from build123d import *

# Parameters (mm, degrees)
BOSS_EXTRUDE1_DEPTH = 3
SKETCH6_W           = 10
SKETCH6_H           = 3
BOSS_EXTRUDE5_DEPTH = 25
SKETCH8_W           = 3
SKETCH8_H           = 10
BOSS_EXTRUDE7_DEPTH = 64.65
SKETCH9_W           = 10
SKETCH9_H           = 3
BOSS_EXTRUDE8_DEPTH = 115.212
SKETCH10_W          = 3
SKETCH10_H          = 22.5
BOSS_EXTRUDE9_DEPTH = 25
SKETCH11_R          = 4
CUT_EXTRUDE1_DEPTH  = 3


with BuildPart() as part:
    # Sketch2 → Boss-Extrude1 (new body)
    with BuildSketch(Plane(origin=(0, 0, 0), x_dir=(1, 0, 0), z_dir=(0, 1, 0))):
        with BuildLine():
            Line((26.055569119, 8.188046441), (26.055569119, -22.834953559))
            Line((26.055569119, -22.834953559), (-26.055569119, -22.834953559))
            Line((-26.055569119, -22.834953559), (-26.055569119, 8.188046441))
            ThreePointArc((-26.055569119, 8.188046441), (-21.514872246, 4.669726518), (-15.870079226, 5.73406431))
            ThreePointArc((-15.870079226, 5.73406431), (-10.616247764, 4.133629141), (-7, 0))
            ThreePointArc((-7, 0), (0, -7), (7, 0))
            ThreePointArc((7, 0), (10.616247764, 4.133629141), (15.870079226, 5.73406431))
            ThreePointArc((15.870079226, 5.73406431), (21.514872246, 4.669726518), (26.055569119, 8.188046441))
        make_face()
    extrude(amount=BOSS_EXTRUDE1_DEPTH)

    # Sketch6 → Boss-Extrude5 (add)
    with BuildSketch(Plane.XY.offset(22.834953559)):
        with Locations((-21.055569119, 1.5)):
            Rectangle(SKETCH6_W, SKETCH6_H)
    extrude(amount=BOSS_EXTRUDE5_DEPTH)

    # Sketch8 → Boss-Extrude7 (add)
    with BuildSketch(Plane(origin=(0, 0, 0), x_dir=(-1, 0, 0), z_dir=(0, -1, 0))):
        with Locations((24.555569119, -42.834953559)):
            Rectangle(SKETCH8_W, SKETCH8_H)
    extrude(amount=BOSS_EXTRUDE7_DEPTH)

    # Sketch9 → Boss-Extrude8 (add)
    with BuildSketch(Plane(origin=(-23.055569119, 0, 0), x_dir=(0, 0, -1), z_dir=(1, 0, 0))):
        with Locations((-42.834953559, -63.15)):
            Rectangle(SKETCH9_W, SKETCH9_H)
    extrude(amount=BOSS_EXTRUDE8_DEPTH)

    # Sketch10 → Boss-Extrude9 (add)
    with BuildSketch(Plane(origin=(0, -61.65, 0), x_dir=(1, 0, 0), z_dir=(0, 1, 0))):
        with Locations((90.656430881, -36.584953559)):
            Rectangle(SKETCH10_W, SKETCH10_H)
    extrude(amount=BOSS_EXTRUDE9_DEPTH)

    # Sketch11 → Cut-Extrude1 (cut)
    with BuildSketch(Plane(origin=(92.156430881, 0, 0), x_dir=(0, 0, -1), z_dir=(1, 0, 0))):
        with Locations((-36.584953559, -49.15)):
            Circle(SKETCH11_R)
    extrude(amount=-CUT_EXTRUDE1_DEPTH, mode=Mode.SUBTRACT)


solid = part.part
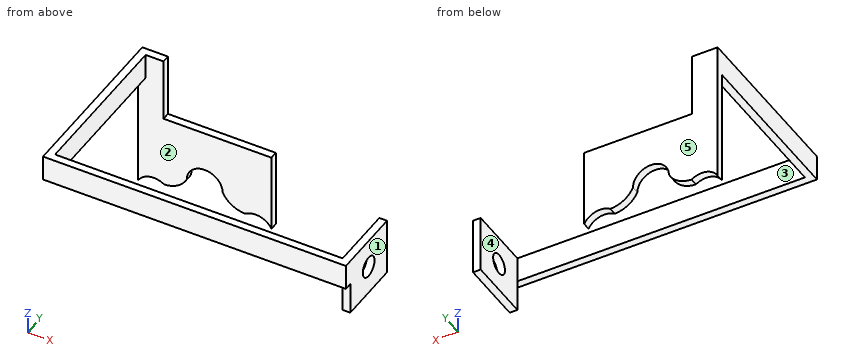
For this review, take the finished solid that the model builds, in its own axes (mm). Face numbers are marked on the shaded views. A direction names the side the tool comes from. Round coordinates to 2 decimals unless told otherwise and drop trailing zeros. Loops run counter-clockwise (first coordinate to the right, second up) from the corner with the lowest first, then second, coordinate; pieces in that order, holes last. Notation, with made-up numbers: (87.5, 26.25) - (122.5, 26.25) arc R24 cw to (122.5, 36.25) - close; hole circle Ø5 at (-15.75, -6.5). An arc over 180 degrees is marked (long way). Answer as CSV lines item,"result".
(1) Tool access review of the marked faces 4 and 5: name each direction out of +Z, -Z, +X, -X, +Y, -Y from which nothing blocks a thin tool from reaching the whole face with its end or side.
Checked values:
face 4,"+Z, -Z, +Y"
face 5,"+Z, -Z, +X, -X, +Y"
(2) Consider section A-A on y = -49.15. Give the boundary of the cut face in (x, z), then the cut area to 3 significant figures.
Checked values:
outline,"(-26.06, 37.83) - (-23.06, 37.83) - (-23.06, 47.83) - (-26.06, 47.83) - close; (89.16, 25.33) - (92.16, 25.33) - (92.16, 32.58) - (89.16, 32.58) - close; (89.16, 40.58) - (92.16, 40.58) - (92.16, 47.83) - (89.16, 47.83) - close"
area,"73.5 mm2"
(3) Consider section D-D on y = -27. Give the boundary of the cut face in (x, z).
Checked values:
outline,"(-26.06, 37.83) - (-23.06, 37.83) - (-23.06, 47.83) - (-26.06, 47.83) - close"
(4) Wall thickness on line 1 (Z direction, x = 90, y = -49); line 2 (X direction, y = -52, z = 44.5); line 3 (Y direction, x = 7, z = 2): over which ranges is each line inside the solid? List them lowest first.
Checked values:
line 1,"z = 25.33 to 32.59, 40.58 to 47.83"
line 2,"x = -26.06 to -23.06, 89.16 to 92.16"
line 3,"y = 0 to 3"
(5) Mouldability with a two-part tool opening along X and no side actions: class the marked faces 1, 2 and 3 as +X half, -X half, draft (parallel to the pull), parting line (faces both ways), or undercut.
Checked values:
face 1,"+X half"
face 2,"draft"
face 3,"undercut"
(6) Insertion check: P1, Ø19.5, axis at x = 3.5, y = -43.5, coming from the -Z side; P2, Ø9, axis at y = -49.15, z = 36.58, coming from the -X side; P3, Ø0.9, axis at x = 90.5, z = 38.5, coming from the +Y side; P4, Ø3.5, axis at x = 91, z = 34, coming from the -Y side. Each pin has a flat end and moves straight along its axis. Give the tip position at first contact, or say it passes through.
Checked values:
P1,"passes through"
P2,"stops at x = -26.06"
P3,"stops at y = -36.65"
P4,"stops at y = -61.65"
(7) Consider section C-C on z = 2. Give the boundary of the cut face in (x, y).
Checked values:
outline,"(-26.06, 0) - (-6.71, 0) - (-6.71, 3) - (-26.06, 3) - close; (6.71, 0) - (26.06, 0) - (26.06, 3) - (6.71, 3) - close"
(8) Consider section B-B on x = 0. Give the boundary of the cut face in (y, z), then the cut area to 3 significant figures.
Checked values:
outline,"(-64.65, 37.83) - (-61.65, 37.83) - (-61.65, 47.83) - (-64.65, 47.83) - close; (0, 7) - (3, 7) - (3, 22.83) - (0, 22.83) - close"
area,"77.5 mm2"
